Can you work these out from the model? Positions are in its coordinate system, mm. Face numbers are marked on the shaded views. Give positions to 0.01 mm unless a question says otherwise; leave off trailing zeros. Order: outer loops, then holes, each group sorted by start corner. A loop starts at its lowest first (then second) coordinate and runs counter-clockwise, first axis right, second up. Notation, with made-up numbers: (-4, 10) - (35, 10) arc R17 ccw to (35, 22) - close; hole circle Ø3 at (71, 32.25). An arc over 180 degrees is marked (long way). Write each question's results on one line, items separated by ' | '. Start each with the question number.
Autodesk Inventor part; units mm, degrees
ref_plane "YZ Plane" through (0, 0, 0) normal (1, 0, 0) x (0, 1, 0)
ref_plane "XZ Plane" through (0, 0, 0) normal (0, 1, 0) x (-1, 0, 0)
ref_plane "XY Plane" through (0, 0, 0) normal (0, 0, 1) x (1, 0, 0)
sketch "Sketch1" plane through (0, 0, 0) normal (0, 0, 1) x (1, 0, 0)
  arc A0 (13.75, 13) -> (18, 8.75) centre (13.75, 8.75) ccw construction
  line L0 (18, -8.75) -> (18, 8.75) construction
  arc A1 (18, -8.75) -> (13.75, -13) centre (13.75, -8.75) ccw construction
  line L1 (-13.75, -13) -> (13.75, -13) construction
  arc A2 (-13.75, -13) -> (-18, -8.75) centre (-13.75, -8.75) ccw construction
  line L2 (-18, 8.75) -> (-18, -8.75) construction
  arc A3 (-18, 8.75) -> (-13.75, 13) centre (-13.75, 8.75) ccw construction
  line L3 (13.75, 13) -> (-13.75, 13) construction
  circle A4 centre (-13.75, 8.75) radius 2.25 construction
  circle A5 centre (13.75, -8.75) radius 2.25 construction
  circle A6 centre (13.75, 8.75) radius 2.25 construction
  circle A7 centre (-13.75, -8.75) radius 2.25 construction
  arc A8 (-20, -11) -> (-16, -15) centre (-16, -11) ccw
  line L4 (16, -15) -> (-16, -15)
  arc A9 (16, -15) -> (20, -11) centre (16, -11) ccw
  line L5 (20, 11) -> (20, -11)
  arc A10 (20, 11) -> (16, 15) centre (16, 11) ccw
  line L6 (-16, 15) -> (16, 15)
  arc A11 (-16, 15) -> (-20, 11) centre (-16, 11) ccw
  line L7 (-20, -11) -> (-20, 11)
  circle A12 centre (-13.75, 8.75) radius 1.75
  circle A13 centre (13.75, 8.75) radius 1.75
  circle A14 centre (13.75, -8.75) radius 1.75
  circle A15 centre (-13.75, -8.75) radius 1.75
  circle A16 centre (0, 0) radius 9.75
  circle A17 centre (-15, 0) radius 2.6
  circle A18 centre (15, 0) radius 2.6
  line L8 (-15, 0) -> (15, 0)
  dimension "d0" = 3.5
  dimension "d1" = 19.5
  dimension "d2" = 5.2
  dimension "d3" = 30
extrude "Extrusion1" add sketch "Sketch1" along normal blind 3
properties part number "button_holder_face"
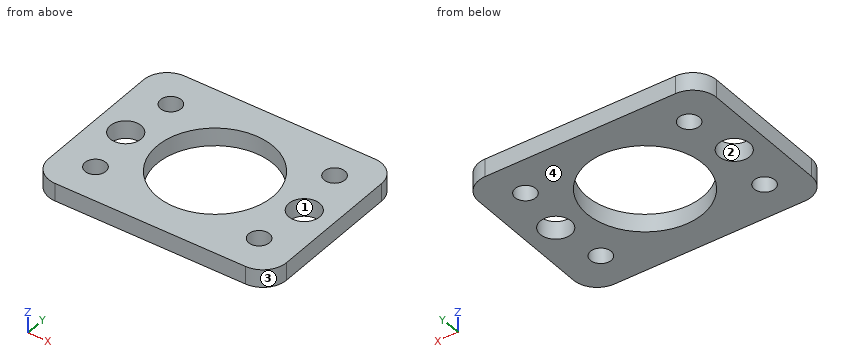
Q1. If we section it at D-D (x = -15): Please give me the cut outline in (y, z), plus the area to 3 significant figures.
Q2. Thinking about a two-plate mould opening in Y: for the marked faces 1, 2, 3 and 4, which applies, released by +Y, released by -Y, zero draft, split by the parting line, or undercut?
Q3. If I drill on probe 1 along Y at (x, z) = (13.75, 1.6); probe 2 along Y at (x, z) = (14.5, 2.75); probe 3 along X at (y, z) = (0.25, 0.7), over which ranges is the centre line in solid material (lowest first)? Write a range as from..to.
Q4. If we section it at C-C (x = 0): Please give me the cut outline in (y, z).
Q5. If we section it at A-A (y = 0): Please give me the cut outline in (x, z).
Q6. If we section it at B-B (z = 1.7): Please give me the cut outline in (x, y).
Findings below:
1) outline: (-15, 0) - (-9.97, 0) - (-9.97, 3) - (-15, 3) - close; (-7.53, 0) - (-2.6, 0) - (-2.6, 3) - (-7.53, 3) - close; (2.6, 0) - (7.53, 0) - (7.53, 3) - (2.6, 3) - close; (9.97, 0) - (15, 0) - (15, 3) - (9.97, 3) - close | area: 59.7 mm2
2) face 1: undercut | face 2: undercut | face 3: released by -Y | face 4: zero draft
3) probe 1: y = -15..-10.5, -7..-2.28, 2.28..7, 10.5..15 | probe 2: y = -15..-10.33, -7.17..-2.55, 2.55..7.17, 10.33..15 | probe 3: x = -20..-17.59, -12.41..-9.75, 9.75..12.41, 17.59..20
4) outline: (-15, 0) - (-9.75, 0) - (-9.75, 3) - (-15, 3) - close; (9.75, 0) - (15, 0) - (15, 3) - (9.75, 3) - close
5) outline: (-20, 0) - (-17.6, 0) - (-17.6, 3) - (-20, 3) - close; (-12.4, 0) - (-9.75, 0) - (-9.75, 3) - (-12.4, 3) - close; (9.75, 0) - (12.4, 0) - (12.4, 3) - (9.75, 3) - close; (17.6, 0) - (20, 0) - (20, 3) - (17.6, 3) - close
6) outline: (-20, -11) arc R4 ccw to (-16, -15) - (16, -15) arc R4 ccw to (20, -11) - (20, 11) arc R4 ccw to (16, 15) - (-16, 15) arc R4 ccw to (-20, 11) - close; hole circle Ø5.2 at (-15, 0); hole circle Ø3.5 at (-13.75, -8.75); hole circle Ø3.5 at (-13.75, 8.75); hole circle Ø19.5 at (0, 0); hole circle Ø3.5 at (13.75, -8.75); hole circle Ø3.5 at (13.75, 8.75); hole circle Ø5.2 at (15, 0)
